For this review, take the finished solid that the model builds, in its own axes (mm). Coordinates: 2 decimals unless noted, no trailing zeros. Order: outer loops, then holes, each group sorted by start corner. A loop starts at its lowest first (then second) coordinate and runs counter-clockwise, first axis right, second up.
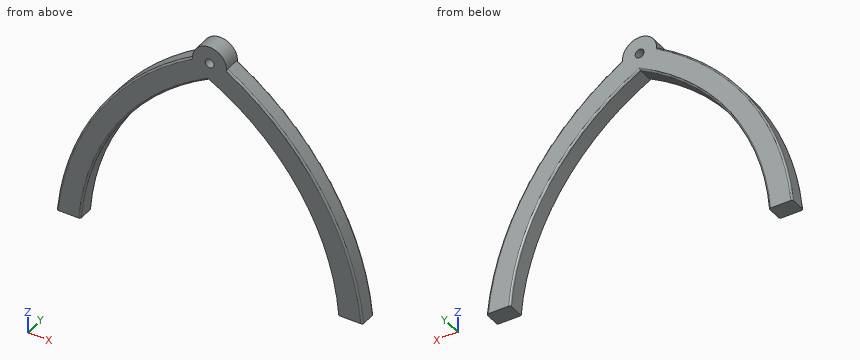
from build123d import *

# Parameters (mm, degrees)
SKETCH_R      = 2.6
EXTRUDE_DEPTH = 5
FILLET_R      = 1


with BuildPart() as part:
    # Sketch → Extrude (new body, symmetric)
    with BuildSketch(Plane.XZ):
        with BuildLine():
            ThreePointArc((10, 0), (0, 10), (-10, 0))
            ThreePointArc((-10, 0), (-64.999628, -52.900238), (-90, -125))
            Line((-76, -125), (-90, -125))
            ThreePointArc((0, -10), (-52.844624, -57.68964), (-76, -125))
            ThreePointArc((76, -125), (52.844624, -57.68964), (0, -10))
            Line((76, -125), (90, -125))
            ThreePointArc((90, -125), (64.999628, -52.900238), (10, 0))
        make_face()
        Circle(SKETCH_R, mode=Mode.SUBTRACT)
    extrude(amount=EXTRUDE_DEPTH, both=True)

    # Fillet
    fillet_edges = [part.edges().sort_by_distance(p)[0] for p in [
        (64.999628, 5, -52.900238),
        (64.999628, -5, -52.900238),
        (-64.999628, 5, -52.900238),
        (-64.999628, -5, -52.900238),
        (-52.844624, 5, -57.68964),
        (-52.844624, -5, -57.68964),
        (52.844624, 5, -57.68964),
    ]]
    fillet(fillet_edges, radius=FILLET_R)


solid = part.part
1. Clearance check with flat-ended pins moving along their axes: pin 1 Ø2 at (y, z) = (0, -56.5) entering from -X; pin 2 Ø2 at (y, z) = (-2, -59) entering from -X; pin 3 Ø4 at (y, z) = (4, -23.5) entering from +X; pin 4 Ø7 at (x, z) = (0, 0) entering from +Y. State where each tip first meets the part, or that it passes through.
Answer below:
pin 1: stops at x = -67.84
pin 2: stops at x = -69.29
pin 3: stops at x = 42.98
pin 4: stops at y = 5
2. Take a section at A-A, the plane y = 1. Give the boundary of the cut face in (x, z).
Answer below:
outline: (-90, -125) - (-76, -125) arc R142.38 cw to (0, -10) arc R142.38 cw to (76, -125) - (90, -125) arc R163.5 ccw to (10, 0) arc R10 ccw to (-10, 0) arc R163.5 ccw to start; hole circle Ø5.2 at (0, 0)
3. To check wall thickness, follow L1, parallel to Z at x = 0, y = -0.25; L2, parallel to X at y = 4.5, z = -103; L3, parallel to X at y = 3.25, z = -95. State the ranges of each line that lie inside material, in increasing order.
Answer below:
L1: z = -10 to -2.6, 2.6 to 10
L2: x = -86.16 to -72.66, 72.66 to 86.16
L3: x = -84.17 to -70.35, 70.35 to 84.17
